Geometry: see drawing. Coordinates: mm, zero at the bounding-box minimum. Coordinates: 2 decimals unless noted, no trailing zeros. Write each loop counter-clockwise with the first axis right and the second up, starting at its lowest first coordinate (ties: lowest second). Pieces come first, ordered by that corner, then holes. Notation, with made-up numbers: (-29.5, 35.25) -> (-4.5, 35.25) arc R25 cw to (-4.5, 73.25) -> close; hole circle Ø5 at (70, -12). An arc over 180 degrees is marked (long way). Use one line per item in the form item = value. Start each with the question number.
(1) First-contact query: pin 1 (2.5 mm diameter, centred on x = 32, y = 23, fed in from -Z); pin 2 (1.4 mm diameter, centred on y = 23, z = 153, fed in from +X); pin 3 (5 mm diameter, centred on x = 41, y = 22, fed in from +Z). Flat tips, straight axial feed; report the tip coordinate or a pass-through.
(2) Ray query, line 1 along Y through (x, z) = (71.5, 137); line 2 along X through (y, z) = (24, 142) (1 decimal); line 3 along X through (y, z) = (8, 130.5) (1 decimal). Return the intervals inside material, ascending.
(3) Cut plane B-B on y = 7. Return the cut outline in (x, z) (1 decimal).
(4) Cut plane C-C on x = 46. Return the cut outline in (y, z) (1 decimal).
(5) Cut plane A-A on z = 174.5. Return the cut outline in (x, y), plus the area to 3 significant figures.
(6) Cut plane D-D on z = 39. Return the cut outline in (x, y).
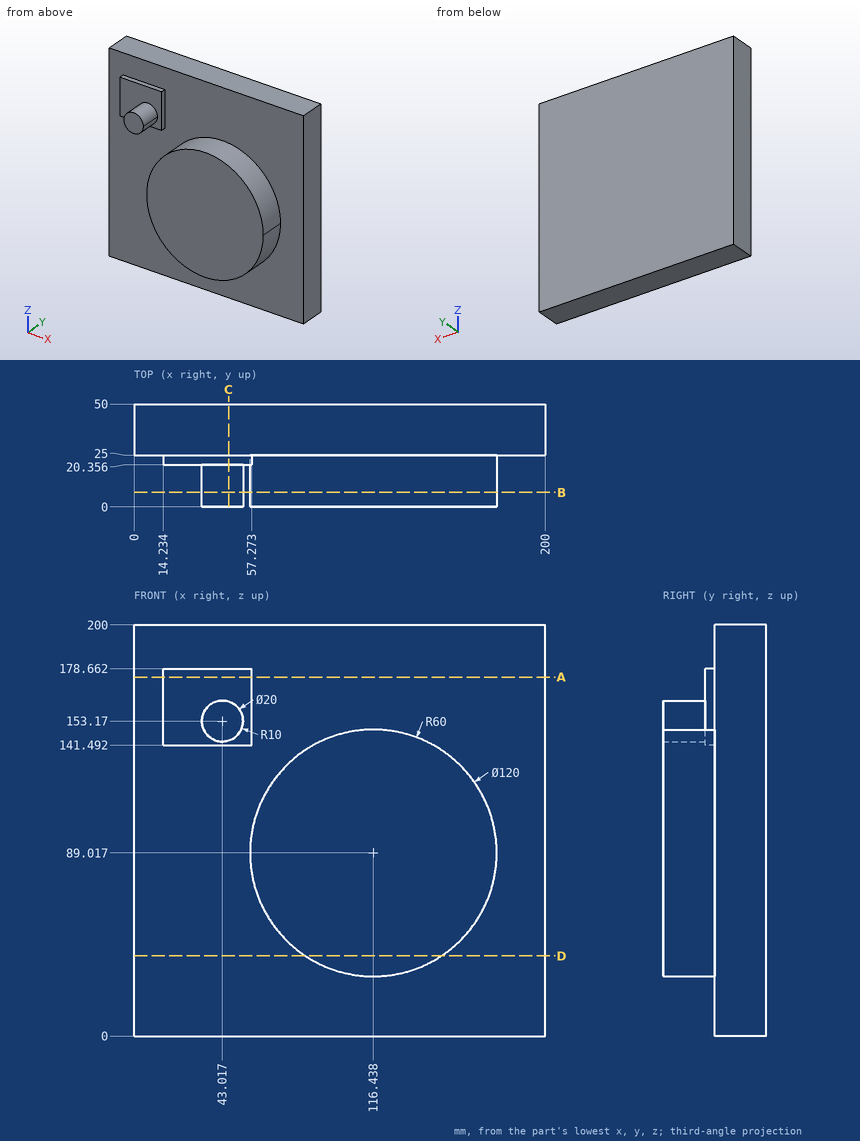
Values:
q1.pin_1 = 141.49
q1.pin_2 = 57.27
q1.pin_3 = 178.66
q2.line_1 = 25 to 50
q2.line_2 = 14.2 to 57.3, 88.3 to 144.6
q2.line_3 = 73.1 to 159.8
q3.outline = (50.5, 146.6) arc R10 ccw to (53, 153.2) arc R10 ccw (long way) to start; circle Ø120 at (116.4, 89)
q4.outline = (0, 143.6) -> (20.4, 143.6) -> (20.4, 141.5) -> (25, 141.5) -> (25, 0) -> (50, 0) -> (50, 200) -> (25, 200) -> (25, 178.7) -> (20.4, 178.7) -> (20.4, 162.7) -> (0, 162.7) -> close
q5.outline = (0, 25) -> (14.23, 25) -> (14.23, 20.36) -> (57.27, 20.36) -> (57.27, 25) -> (200, 25) -> (200, 50) -> (0, 50) -> close
q5.area = 5,200 mm2
q6.outline = (0, 25) -> (83.3, 25) -> (83.3, 0) -> (149.58, 0) -> (149.58, 25) -> (200, 25) -> (200, 50) -> (0, 50) -> close
